from build123d import *

# Parameters (mm, degrees)
SKETCH1_W           = 11.63
SKETCH1_H           = 2.41
BOSS_EXTRUDE1_DEPTH = 2.92
SKETCH2_R           = 0.25
BOSS_EXTRUDE2_DEPTH = 2.315
SKETCH3_R           = 0.25
BOSS_EXTRUDE3_DEPTH = 2.315


with BuildPart() as part:
    # Sketch1 → Boss-Extrude1 (new body)
    with BuildSketch(Plane(origin=(0, 0, 0), x_dir=(1, 0, 0), z_dir=(0, 1, 0))):
        with Locations((5.815, 1.205)):
            Rectangle(SKETCH1_W, SKETCH1_H)
    extrude(amount=BOSS_EXTRUDE1_DEPTH)

    # Sketch2 → Boss-Extrude2 (add)
    with BuildSketch(Plane(origin=(11.63, 0, 0), x_dir=(0, 0, -1), z_dir=(1, 0, 0))):
        with Locations((1.167158441, 1.465733238)):
            Circle(SKETCH2_R)
    extrude(amount=BOSS_EXTRUDE2_DEPTH)

    # Sketch3 → Boss-Extrude3 (add)
    with BuildSketch(Plane.ZY):
        with Locations((-1.201708257, 1.412791091)):
            Circle(SKETCH3_R)
    extrude(amount=BOSS_EXTRUDE3_DEPTH)


solid = part.part
Input: part model. Units: mm. Frame: model coordinates. Coordinates: 2 decimals unless noted, no trailing zeros. Order: outer loops, then holes, each group sorted by start corner. A loop starts at its lowest first (then second) coordinate and runs counter-clockwise, first axis right, second up.
1. Cut plane B-B, the plane y = 2.35. Return loops of the section in (x, z).
Checked values:
outline: (0, -2.41) - (11.63, -2.41) - (11.63, 0) - (0, 0) - close
2. Contact query for flat-ended pins moving along their axis: P1, Ø1, axis at x = 7.5, y = 2, coming from the +Z side; P2, Ø1, axis at y = 1.5, z = -2, coming from the -X side. Output: stop coordinate, or through.
Checked values:
P1: stops at z = 0
P2: stops at x = 0
3. Ray query, line 1 along X through (y, z) = (0.8, -2.3); line 2 along Y through (x, z) = (-0.5, -1.3). Return the intervals inside material, ascending.
Checked values:
line 1: x = 0 to 11.63
line 2: y = 1.18 to 1.64
4. Cut plane A-A, the plane z = -1.25. Return loops of the section in (x, y) (1 decimal).
Checked values:
outline: (-2.3, 1.2) - (0, 1.2) - (0, 0) - (11.6, 0) - (11.6, 1.2) - (13.9, 1.2) - (13.9, 1.7) - (11.6, 1.7) - (11.6, 2.9) - (0, 2.9) - (0, 1.7) - (-2.3, 1.7) - close
